from build123d import *

# Parameters (mm, degrees)
SKETCH1_R           = 8.4
BOSS_EXTRUDE1_DEPTH = 30
SKETCH3_R           = 10
BOSS_EXTRUDE2_DEPTH = 1
BOSS_EXTRUDE3_DEPTH = 10
BOSS_EXTRUDE4_DEPTH = 30
CUT_EXTRUDE1_DEPTH  = 66
CHAMFER1_SIZE       = 1.5
SKETCH7_R           = 1.5
SKETCH7_R_2         = 2.5
CUT_EXTRUDE2_DEPTH  = 42


with BuildPart() as part:
    # Sketch1 → Boss-Extrude1 (new body)
    with BuildSketch(Plane.XY):
        Circle(SKETCH1_R)
    extrude(amount=BOSS_EXTRUDE1_DEPTH)

    # Sketch3 → Boss-Extrude2 (add)
    with BuildSketch(Plane.XY.offset(30)):
        Circle(SKETCH3_R)
    extrude(amount=BOSS_EXTRUDE2_DEPTH)

    # Sketch4 → Boss-Extrude3 (add)
    with BuildSketch(Plane.XY.offset(31)):
        with BuildLine():
            Line((0, 15), (105, 15))
            Line((105, 15), (105, -15))
            Line((105, -15), (0, -15))
            ThreePointArc((0, -15), (-15, 0), (0, 15))
        make_face()
    extrude(amount=BOSS_EXTRUDE3_DEPTH)

    # Sketch5 → Boss-Extrude4 (add)
    with BuildSketch(Plane(origin=(0, 15, 0), x_dir=(1, 0, 0), z_dir=(0, 1, 0))):
        with BuildLine():
            Line((40, -31), (105, -31))
            Line((105, -31), (105, -11))
            Line((105, -11), (50, -11))
            ThreePointArc((50, -11), (46.464466094, -12.464466094), (45, -16))
            Line((45, -16), (45, -26))
            ThreePointArc((45, -26), (43.535533906, -29.535533906), (40, -31))
        make_face()
    extrude(amount=-BOSS_EXTRUDE4_DEPTH)

    # Sketch6 → Cut-Extrude1 (cut)
    with BuildSketch(Plane(origin=(105, 0, 0), x_dir=(0, 0, -1), z_dir=(1, 0, 0))):
        with BuildLine():
            Line((-23.197056275, 4.553712276), (-28.802943725, 4.553712276))
            Line((-28.802943725, 4.553712276), (-30.710050506, 6.460819058))
            Line((-30.710050506, 6.460819058), (-30.710050506, 7.753712276))
            Line((-30.710050506, 7.753712276), (-29.482842712, 7.753712276))
            ThreePointArc((-29.482842712, 7.753712276), (-28.83612704, 8.185833874), (-28.987867966, 8.948687023))
            Line((-28.987867966, 8.948687023), (-30.387867966, 10.348687023))
            Line((-30.387867966, 10.348687023), (-36.294974747, 10.348687023))
            Line((-36.294974747, 10.348687023), (-36.294974747, 4.441580242))
            Line((-36.294974747, 4.441580242), (-34.894974747, 3.041580242))
            ThreePointArc((-34.894974747, 3.041580242), (-34.132121597, 2.889839316), (-33.7, 3.536554989))
            Line((-33.7, 3.536554989), (-33.7, 4.763762783))
            Line((-33.7, 4.763762783), (-32.407106781, 4.763762783))
            Line((-32.407106781, 4.763762783), (-30.5, 2.856656002))
            Line((-30.5, 2.856656002), (-30.5, -2.749231449))
            Line((-30.5, -2.749231449), (-32.407106781, -4.65633823))
            Line((-32.407106781, -4.65633823), (-33.7, -4.65633823))
            Line((-33.7, -4.65633823), (-33.7, -3.429130436))
            ThreePointArc((-33.7, -3.429130436), (-34.132121597, -2.782414763), (-34.894974747, -2.934155689))
            Line((-34.894974747, -2.934155689), (-36.294974747, -4.334155689))
            Line((-36.294974747, -4.334155689), (-36.294974747, -10.24126247))
            Line((-36.294974747, -10.24126247), (-30.387867966, -10.24126247))
            Line((-30.387867966, -10.24126247), (-28.987867966, -8.84126247))
            ThreePointArc((-28.987867966, -8.84126247), (-28.83612704, -8.078409321), (-29.482842712, -7.646287724))
            Line((-29.482842712, -7.646287724), (-30.710050506, -7.646287724))
            Line((-30.710050506, -7.646287724), (-30.710050506, -6.353394505))
            Line((-30.710050506, -6.353394505), (-28.802943725, -4.446287724))
            Line((-28.802943725, -4.446287724), (-23.197056275, -4.446287724))
            Line((-23.197056275, -4.446287724), (-21.289949494, -6.353394505))
            Line((-21.289949494, -6.353394505), (-21.289949494, -7.646287724))
            Line((-21.289949494, -7.646287724), (-22.517157288, -7.646287724))
            ThreePointArc((-22.517157288, -7.646287724), (-23.16387296, -8.078409321), (-23.012132034, -8.84126247))
            Line((-23.012132034, -8.84126247), (-21.612132034, -10.24126247))
            Line((-21.612132034, -10.24126247), (-15.705025253, -10.24126247))
            Line((-15.705025253, -10.24126247), (-15.705025253, -4.334155689))
            Line((-15.705025253, -4.334155689), (-17.105025253, -2.934155689))
            ThreePointArc((-17.105025253, -2.934155689), (-17.867878403, -2.782414763), (-18.3, -3.429130436))
            Line((-18.3, -3.429130436), (-18.3, -4.65633823))
            Line((-18.3, -4.65633823), (-19.592893219, -4.65633823))
            Line((-19.592893219, -4.65633823), (-21.5, -2.749231449))
            Line((-21.5, -2.749231449), (-21.5, 2.856656002))
            Line((-21.5, 2.856656002), (-19.592893219, 4.763762783))
            Line((-19.592893219, 4.763762783), (-18.3, 4.763762783))
            Line((-18.3, 4.763762783), (-18.3, 3.536554989))
            ThreePointArc((-18.3, 3.536554989), (-17.867878403, 2.889839316), (-17.105025253, 3.041580242))
            Line((-17.105025253, 3.041580242), (-15.705025253, 4.441580242))
            Line((-15.705025253, 4.441580242), (-15.705025253, 10.348687023))
            Line((-15.705025253, 10.348687023), (-21.612132034, 10.348687023))
            Line((-21.612132034, 10.348687023), (-23.012132034, 8.948687023))
            ThreePointArc((-23.012132034, 8.948687023), (-23.16387296, 8.185833874), (-22.517157288, 7.753712276))
            Line((-22.517157288, 7.753712276), (-21.289949494, 7.753712276))
            Line((-21.289949494, 7.753712276), (-21.289949494, 6.460819058))
            Line((-21.289949494, 6.460819058), (-23.197056275, 4.553712276))
        make_face()
    extrude(amount=-CUT_EXTRUDE1_DEPTH, mode=Mode.SUBTRACT)

    # Chamfer1
    chamfer1_edges = [part.edges().sort_by_distance(p)[0] for p in [
        (-15, 0, 31),
        (20, -15, 31),
        (-15, 0, 41),
        (52.5, -15, 41),
        (52.5, 15, 41),
        (20, 15, 31),
        (43.535533906, -15, 29.535533906),
        (45, -15, 21),
        (46.464466094, -15, 12.464466094),
        (77.5, -15, 11),
        (77.5, 15, 11),
        (46.464466094, 15, 12.464466094),
        (45, 15, 21),
        (43.535533906, 15, 29.535533906),
    ]]
    chamfer(chamfer1_edges, length=CHAMFER1_SIZE)

    # Sketch7 → Cut-Extrude2 (cut, through all)
    with BuildSketch(Plane.XY.offset(41)):
        with Locations((53, 0)):
            Circle(SKETCH7_R)
        with Locations((79, 0)):
            Circle(SKETCH7_R)
        with Locations((98.6, 0)):
            Circle(SKETCH7_R_2)
        Circle(SKETCH7_R_2)
    extrude(amount=-CUT_EXTRUDE2_DEPTH, mode=Mode.SUBTRACT)


solid = part.part
Geometry check sheet. Reference: the model listing, model coordinates, mm. A direction names the side the tool comes from. Coordinates: 2 decimals unless noted, no trailing zeros. Order: outer loops, then holes, each group sorted by start corner. A loop starts at its lowest first (then second) coordinate and runs counter-clockwise, first axis right, second up. Notation, with made-up numbers: (28.5, -32) - (68.5, -32) arc R22 ccw to (68.5, 3) - close; hole circle Ø7 at (83.5, 64). An arc over 180 degrees is marked (long way). One line per item, written item: value.
(1) Sectioned sample at B-B (y = 0). Count the separate pieces of the cut face and the enclosed holes in it, and give its area (3 significant figures).
Data:
separate pieces: 9
enclosed holes: 0
area: 1,940 mm^2
(2) Thickness scan on probe 1 along Y at (x, z) = (81, 33); probe 2 along Y at (x, z) = (98.6, 19); probe 3 along Y at (x, z) = (53, 33.25). Record the ranges inside material, lowest first. Write a range as from..to.
Data:
probe 1: y = -15..-10.24, -4.66..4.76, 10.35..15
probe 2: y = -15..-10.24, -4.66..-2.5, 2.5..4.76, 10.35..15
probe 3: y = -15..-10.24, -4.66..-1.5, 1.5..4.76, 10.35..15
(3) Access from +Z, -Z, +X, -X, +Y, -Y to the whole of each face (thin tool, end or side, straight path). Record for faces 1 (the face through (41.13, 0.1, 30.87)), 2 (the face through (-5, 7, 30)), 3 (the face through (78, 3, 11)), 4 (the face through (72, 7, 36.295)).
Data:
face 1: -Z, +Y, -Y
face 2: -Z
face 3: -Z, +X, +Y, -Y
face 4: +X
(4) Sectioned sample at D-D (z = 6). Enter the section's corners in (x, y), and give its area (3 significant figures).
Data:
outline: circle Ø16.8 at (0, 0); hole circle Ø5 at (0, 0)
area: 202 mm^2
(5) Sectioned sample at A-A (x = 34). Enter the section's corners in (y, z).
Data:
outline: (-15, 32.5) - (-13.5, 31) - (13.5, 31) - (15, 32.5) - (15, 39.5) - (13.5, 41) - (-13.5, 41) - (-15, 39.5) - close
(6) Release check for a two-part mould opening along X. For faces 5 (the face through (105, 0, 20)), 6 (the face through (75, 10.349, 19)), 7 (the face through (-0.54, -2.44, 20.79)) record: +X half, -X half, draft (parallel to the pull), parting line (faces both ways), or undercut.
Data:
face 5: +X half
face 6: draft
face 7: undercut
(7) Depth check by flat-ended pin: pin 1 Ø1.6 at (y, z) = (5.5, 34.5) entering from +X; pin 2 Ø4 at (x, y) = (53, 0) entering from +Z; pin 3 Ø1.8 at (x, y) = (69, -6) entering from -Z; pin 4 Ø4 at (y, z) = (-5, 29.5) entering from -X. Enter the tip coordinate at first touch or a pass-through.
Data:
pin 1: stops at x = 39
pin 2: stops at z = 41
pin 3: stops at z = 11
pin 4: stops at x = -13.19
